Build history of the part. All positions in model axes, mm. Face numbers are marked on the shaded views. Round coordinates to 2 decimals unless told otherwise and drop trailing zeros. Write each loop counter-clockwise with the first axis right and the second up, starting at its lowest first coordinate (ties: lowest second). Pieces come first, ordered by that corner, then holes.
Item 1: Band-saw the part on B-B, the plane x = 17.5. Write the cut outline in (y, z), then the cut area to 3 significant figures.
Item 2: Band-saw the part on A-A, the plane z = 4. Write the cut outline in (x, y), then the cut area to 3 significant figures.
Item 3: Mould opens along Y. For the marked faces 1 and 2 say: +Y half, -Y half, draft (parallel to the pull), parting line (faces both ways), or undercut.
Item 4: Wall check: probe 1 along Y at (x, z) = (-27.5, 6.5); probe 2 along Y at (x, z) = (17.5, -0.75); probe 3 along Z at (x, y) = (0, 19). Give the ranges that are in metal, low to high.
Item 5: Band-saw the part on C-C, the plane y = 0. Write the cut outline in (x, z).
Item 6: Band-saw the part on D-D, the plane y = 4.5. Write the cut outline in (x, z).
Item 7: Drop flat-ended pins along their axis: pin 1 Ø0.8 at (x, y) = (28, 16) entering from +Z; pin 2 Ø1 at (x, z) = (-25, 4) entering from +Y. Give the stop position or say it passes through.
Autodesk Fusion 360 part; units mm, degrees
sketch "Sketch1" plane through (0, 0, 0) normal (0, 0, 1) x (1, 0, 0)
  line L0 (27.5, 16.5) -> (-27.5, 16.5) construction
  line L1 (-27.5, 16.5) -> (-27.5, -16.5) construction
  line L2 (-27.5, -16.5) -> (27.5, -16.5) construction
  line L3 (27.5, -16.5) -> (27.5, 16.5) construction
  line L4 (27.5, 16.5) -> (-27.5, -16.5) construction
  line L5 (-27.5, 16.5) -> (27.5, -16.5) construction
  line L6 (-29.5, 21.5) -> (29.5, 21.5)
  line L7 (32.5, 18.5) -> (32.5, -18.5)
  line L8 (29.5, -21.5) -> (-29.5, -21.5)
  line L9 (-32.5, -18.5) -> (-32.5, 18.5)
  line L10 (-32.5, 21.5) -> (32.5, -21.5) construction
  line L11 (32.5, 21.5) -> (-32.5, -21.5) construction
  arc A0 (-29.5, 21.5) -> (-32.5, 18.5) centre (-29.5, 18.5) ccw
  arc A1 (-32.5, -18.5) -> (-29.5, -21.5) centre (-29.5, -18.5) ccw
  arc A2 (29.5, -21.5) -> (32.5, -18.5) centre (29.5, -18.5) ccw
  arc A3 (32.5, 18.5) -> (29.5, 21.5) centre (29.5, 18.5) ccw
  circle A4 centre (27.5, -16.5) radius 3
  circle A5 centre (27.5, -16.5) radius 1.264
  circle A6 centre (27.5, 16.5) radius 3
  circle A7 centre (27.5, 16.5) radius 1.264
  circle A8 centre (-27.5, -16.5) radius 3
  circle A9 centre (-27.5, -16.5) radius 1.264
  circle A10 centre (-27.5, 16.5) radius 3
  circle A11 centre (-27.5, 16.5) radius 1.264
  circle A12 centre (17.5, 0) radius 1.5
  circle A13 centre (-17.5, 0) radius 1.5
  dimension "d1" = 55
  dimension "d2" = 33
  dimension "d3" = 65
  dimension "d4" = 43
  dimension "d5" = 3
  dimension "d6" = 6
  dimension "d7" = 2.528
  dimension "d8" = 6
  dimension "d9" = 2.528
  dimension "d10" = 2.528
  dimension "d11" = 6
  dimension "d12" = 2.528
  dimension "d13" = 6
  dimension "d14" = 17.5
  dimension "d15" = 3
  dimension "d16" = 17.5
  dimension "d17" = 3
extrude "Extrude1" add sketch "Sketch1" against normal blind 2 contours L6 L7 L8 L9 A0 A1 A2 A3 | A4 | A5 | A6 | A7 | A8 | A9 | A10 | A11
extrude "Extrude2" add sketch "Sketch1" along normal blind 8 contours A4 | A6 | A8 | A10
fillet "Fillet1" radius 2 4 edges at (-30.297, 17.5848, 0) (-30.297, -15.4152, 0) (24.703, -15.4152, 0) (24.703, 17.5848, 0)
equation "d7 = ( 1.264 * 2 ) * 1 mm"
equation "d8 = d6"
equation "d9 = d7"
equation "d10 = d7"
equation "d11 = d6"
equation "d12 = d7"
equation "d13 = d6"
equation "d14 = ( 35 / 2 ) * 1 mm"
equation "d16 = d14"
equation "d17 = d15"
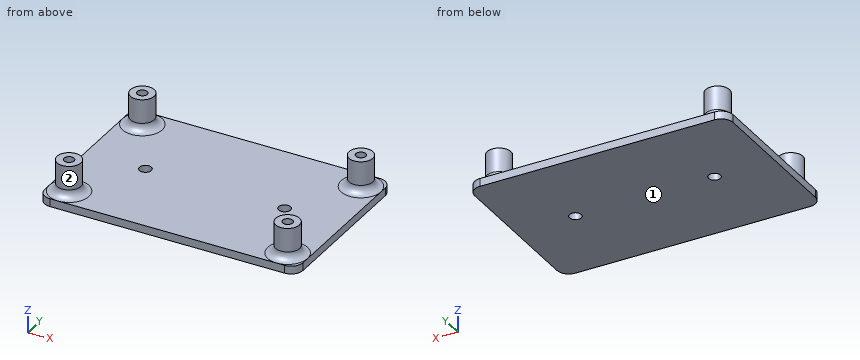
Results:
1. outline: (-21.5, -2) - (-1.5, -2) - (-1.5, 0) - (-21.5, 0) - close; (1.5, -2) - (21.5, -2) - (21.5, 0) - (1.5, 0) - close
1. area: 80.0 mm2
2. outline: circle Ø6 at (-27.5, -16.5); circle Ø6 at (-27.5, 16.5); circle Ø6 at (27.5, -16.5); circle Ø6 at (27.5, 16.5); hole circle Ø2.53 at (-27.5, -16.5); hole circle Ø2.53 at (-27.5, 16.5); hole circle Ø2.53 at (27.5, -16.5); hole circle Ø2.53 at (27.5, 16.5)
2. area: 93.0 mm2
3. face 1: draft
3. face 2: undercut
4. probe 1: y = -19.5 to -17.76, -15.24 to -13.5, 13.5 to 15.24, 17.76 to 19.5
4. probe 2: y = -21.5 to -1.5, 1.5 to 21.5
4. probe 3: z = -2 to 0
5. outline: (-32.5, -2) - (-19, -2) - (-19, 0) - (-32.5, 0) - close; (-16, -2) - (16, -2) - (16, 0) - (-16, 0) - close; (19, -2) - (32.5, -2) - (32.5, 0) - (19, 0) - close
6. outline: (-32.5, -2) - (32.5, -2) - (32.5, 0) - (-32.5, 0) - close
7. pin 1: stops at z = 0
7. pin 2: stops at y = 18.74
